Study the drawing (mm; zero at the part's minimum x, y, z) and answer. Coordinates: 2 decimals unless noted, no trailing zeros. Loops run counter-clockwise (first coordinate to the right, second up) from the corner with the lowest first, then second, coordinate; pieces in that order, holes last. Notation, with made-up numbers: (-33.75, 67.25) -> (-9.75, 67.25) arc R25 cw to (-9.75, 94.25) -> close; hole circle Ø6 at (-21, 74). An arc over 180 degrees is marked (long way). Answer as a JSON object with one key per item and string values. Group by question number.
Q1. The part is cut by section C-C on y = 145. Write down the section's boundary in (x, z), and give its area (3 significant figures).
Q2. Straight lines are drawn through the part: line 1 along Y through (x, z) = (22.5, 10.75); line 2 along X through (y, z) = (119.5, 12.5); line 3 along Z through (x, y) = (23, 119.5). For each, find the intervals that lie inside material, in ascending order. Write a range as [from, to].
Q3. Each of these flat-tipped pins is pushed along its axis until it touches: P1, Ø2.5, axis at y = 3, z = 18, coming from the +X side; P2, Ø12, axis at y = 84, z = 20, coming from the +X side; P3, Ø2.5, axis at y = 3.5, z = 10, coming from the -X side. Where does it stop, or does it pass through?
Q4. The part is cut by section A-A on x = 22.5. Write down the section's boundary in (y, z).
Q5. The part is cut by section D-D on z = 1.5. Write down the section's boundary in (x, y), and give its area (3 significant figures).
Q6. The part is cut by section B-B on z = 12.5. Write down the section's boundary in (x, y).
Q7. Determine the mould class of the marked faces 1 and 2 for opening direction Y: released by +Y, released by -Y, zero draft, split by the parting line, or undercut.
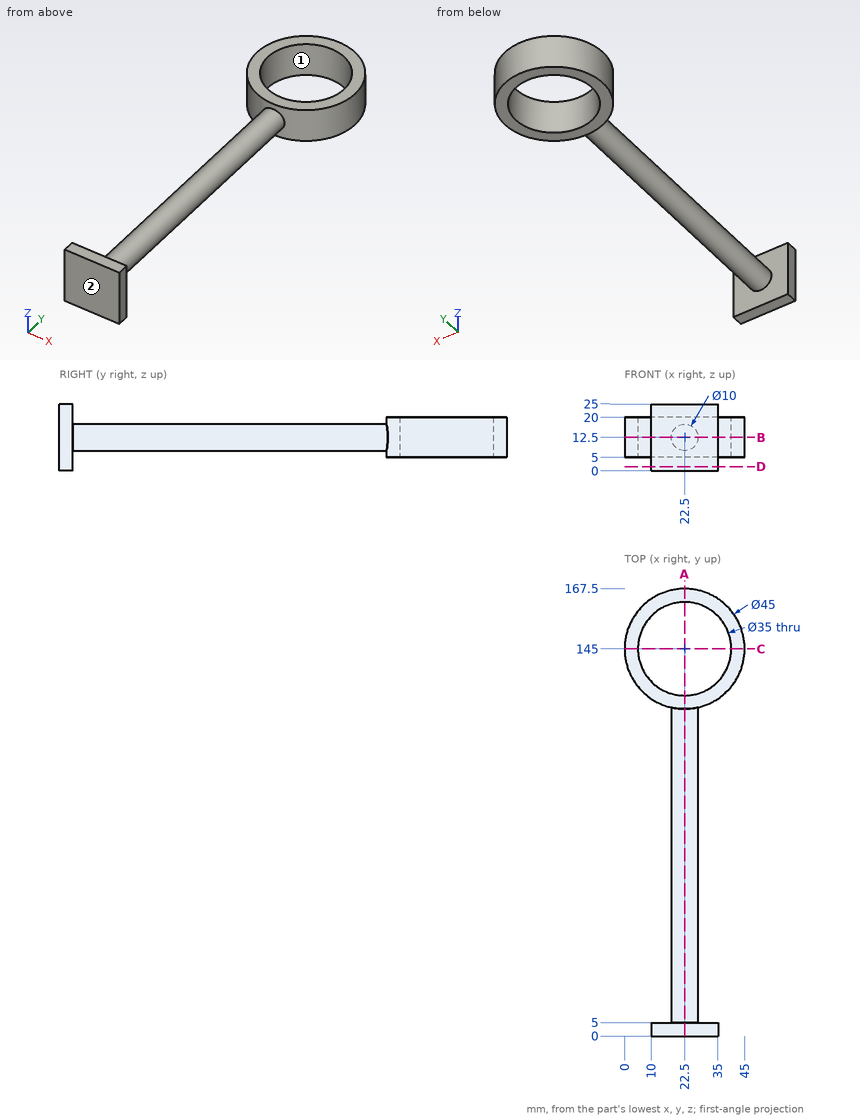
Final values:
{
 "1": {"outline": "(0, 5) -> (5, 5) -> (5, 20) -> (0, 20) -> close; (40, 5) -> (45, 5) -> (45, 20) -> (40, 20) -> close", "area": "150 mm2"},
 "2": {"line 1": "y = [0, 127.5], [162.5, 167.5]", "line 2": "x = [17.5, 27.5]", "line 3": "z = [7.53, 17.47]"},
 "3": {"P1": "stops at x = 35", "P2": "stops at x = 27.27", "P3": "stops at x = 10"},
 "4": {"outline": "(0, 0) -> (5, 0) -> (5, 7.5) -> (122.5, 7.5) -> (122.5, 5) -> (127.5, 5) -> (127.5, 20) -> (122.5, 20) -> (122.5, 17.5) -> (5, 17.5) -> (5, 25) -> (0, 25) -> close; (162.5, 5) -> (167.5, 5) -> (167.5, 20) -> (162.5, 20) -> close"},
 "5": {"outline": "(10, 0) -> (35, 0) -> (35, 5) -> (10, 5) -> close", "area": "125 mm2"},
 "6": {"outline": "(10, 0) -> (35, 0) -> (35, 5) -> (27.5, 5) -> (27.5, 123.06) arc R22.5 ccw (long way) to (17.5, 123.06) -> (17.5, 5) -> (10, 5) -> close; hole circle Ø35 at (22.5, 145)"},
 "7": {"face 1": "undercut", "face 2": "released by -Y"}
}
